Geometry check sheet. Reference: the model listing, model coordinates, mm. Coordinates: 2 decimals unless noted, no trailing zeros. Write each loop counter-clockwise with the first axis right and the second up, starting at its lowest first coordinate (ties: lowest second). Pieces come first, ordered by that corner, then holes. Notation, with made-up numbers: (-35.5, -40) -> (3.5, -40) arc R26 ccw to (3.5, -21) -> close; hole circle Ø10 at (-35.75, 89.5). An arc over 180 degrees is marked (long way). Use a Markdown table: item, result.
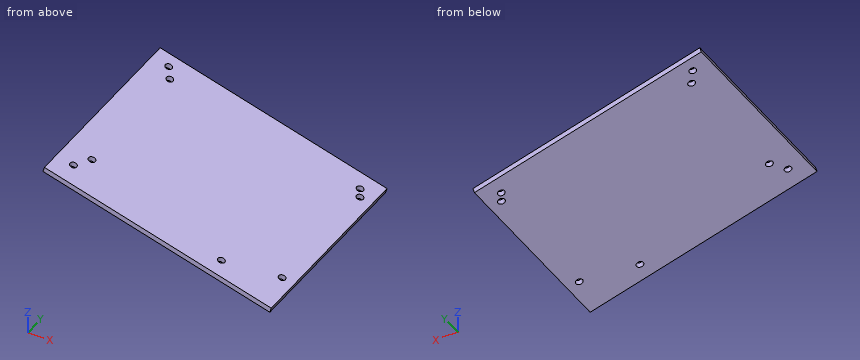
Autodesk Inventor part; units mm, degrees
ref_plane "YZ Plane" through (0, 0, 0) normal (1, 0, 0) x (0, 1, 0)
ref_plane "XZ Plane" through (0, 0, 0) normal (0, 1, 0) x (-1, 0, 0)
ref_plane "XY Plane" through (0, 0, 0) normal (0, 0, 1) x (1, 0, 0)
ref_plane "Work Plane1" through (208.4454, -9.6874, 112.9362) normal (0.2714244, 0, 0.9624598) x (0.9624598, 0, -0.2714244)
sketch "Sketch1" plane through (208.4454, -9.6874, 112.9362) normal (0.2714244, 0, 0.9624598) x (0.9624598, 0, -0.2714244)
  line L0 (-398.5087, 80.1361) -> (-262.5087, 80.1361)
  line L1 (-262.5087, 80.1361) -> (-262.5087, -32.8639)
  line L2 (-262.5087, -32.8639) -> (-398.5087, -32.8639)
  line L3 (-398.5087, -32.8639) -> (-398.5087, 80.1361)
  circle A0 centre (-388.5087, 72.1361) radius 2
  circle A1 centre (-272.5087, 70.1361) radius 2
  circle A2 centre (-298.5087, -22.8639) radius 2
  circle A3 centre (-388.5087, -20.8639) radius 2
  line L4 (-383.5087, -10.8639) -> (-269.5087, -10.8639)
  line L5 (-269.5087, -10.8639) -> (-269.5087, 65.1361)
  line L6 (-269.5087, 65.1361) -> (-383.5087, 65.1361)
  line L7 (-383.5087, 65.1361) -> (-383.5087, -10.8639)
  circle A4 centre (-383.5087, -10.8639) radius 2
  circle A5 centre (-269.5087, -10.8639) radius 2
  circle A6 centre (-269.5087, 65.1361) radius 2
  circle A7 centre (-383.5087, 65.1361) radius 2
  point P0 (-169.9666, 9.6874)
  dimension "d0" = 136
  dimension "d1" = 113
  dimension "d2" = 4
  dimension "d3" = 4
  dimension "d4" = 4
  dimension "d5" = 4
  dimension "d6" = 116
  dimension "d7" = 93
  dimension "d8" = 93
  dimension "d9" = 90
  dimension "d10" = 10
  dimension "d11" = 10
  dimension "d12" = 0
  dimension "d13" = 114
  dimension "d14" = 76
  dimension "d15" = 15
  dimension "d16" = 15
  dimension "d17" = 4
  dimension "d18" = 4
  dimension "d19" = 4
  dimension "d20" = 4
extrude "Extrusion1" add sketch "Sketch1" along normal blind 3 contours L0 L1 L2 L3 | L7 A4 L4 | A4 L7 A7 L6 A6 L5 A5 L4 | A5 L5 L4 | L7 L6 A7 | A6 L6 L5 picked at (-383.0711, -9.6133) picked at (-269.9463, -9.6133) picked at (-383.0711, 63.8855) picked at (-269.9463, 63.8855)
extrude "Extrusion2" cut sketch "Sketch1" along normal through all contours L7 A4 L4 | L4 A4 L7 | A5 L5 L4 | L4 L5 A5 | A7 L6 L7 | L7 L6 A7 | A6 L6 L5 | L5 L6 A6
equation "\"d3\" = d2"
equation "\"d4\" = d2"
equation "\"d5\" = d4"
equation "\"d17\" = d4"
equation "\"d18\" = d4"
equation "\"d19\" = d17"
equation "\"d20\" = d18"
properties part number "SpartanLap"
Item 1: Section check B-B on z = 212.5. Record the boundary of the cut face in (x, y), then the cut area to 3 significant figures.
Answer block:
| item | result |
|---|---|
| outline | (-144.6, -42.55) -> (-133.55, -42.55) -> (-133.55, 70.45) -> (-144.6, 70.45) -> close |
| area | 1,250 mm^2 |
Item 2: Thickness scan on L1, parallel to Z at x = -146, y = 48.5; L2, parallel to Z at x = -118, y = 20.5. Record the ranges inside material, lowest first. Write a range as [from, to].
Answer block:
| item | result |
|---|---|
| L1 | z = [212.89, 216.01] |
| L2 | z = [205, 208.11] |
Item 3: Section check A-A on y = 9.5. Record the boundary of the cut face in (x, z).
Answer block:
| item | result |
|---|---|
| outline | (-175.1, 221.1) -> (-44.21, 184.19) -> (-43.39, 187.07) -> (-174.29, 223.99) -> close |
Item 4: Depth check by flat-ended pin: P1, Ø4, axis at x = -150, y = 15.5, coming from the -Z side; P2, Ø12, axis at y = -12, z = 217, coming from the -X side; P3, Ø2, axis at x = -68, y = -10, coming from the -Z side. Enter the tip coordinate at first touch or a pass-through.
Answer block:
| item | result |
|---|---|
| P1 | stops at z = 213.46 |
| P2 | stops at x = -175.1 |
| P3 | stops at z = 190.61 |
